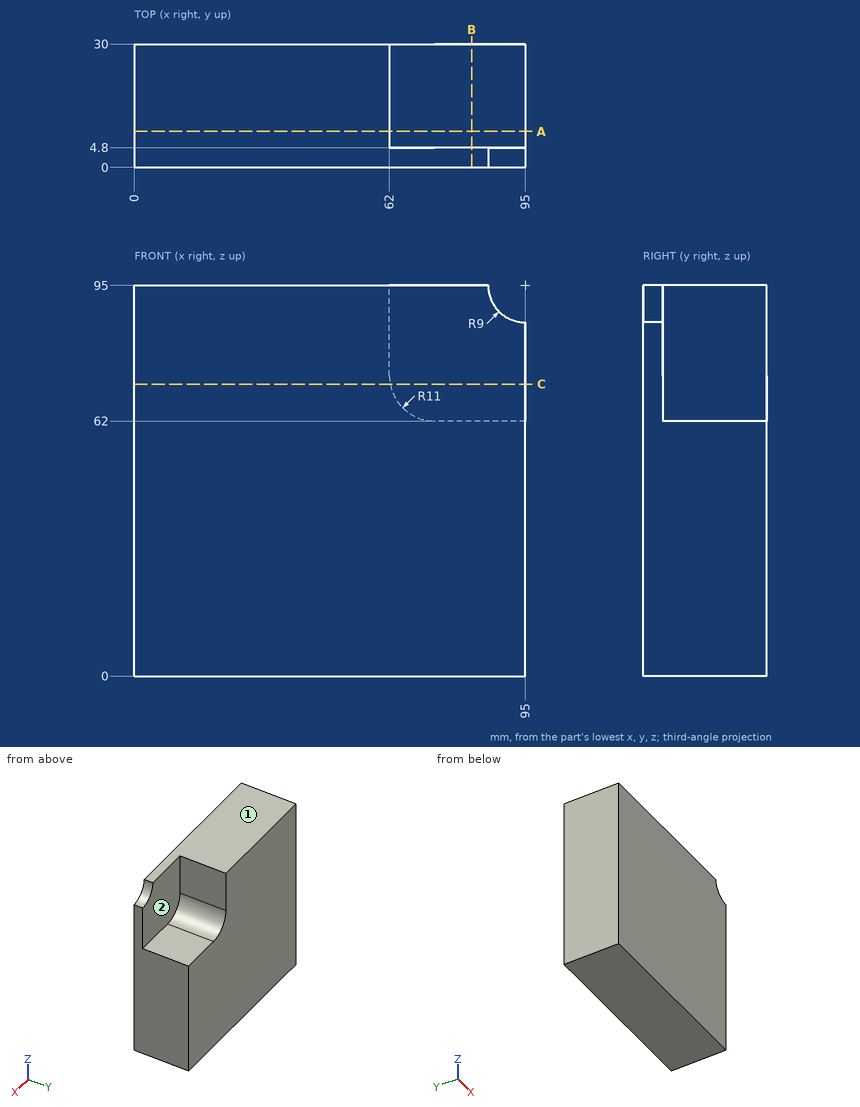
For this review, use the dimensioned drawing (mm, ordinates from the lowest corner) and the shaded views. A direction names the side the tool comes from. Round coordinates to 2 decimals unless told otherwise and drop trailing zeros. Write each loop counter-clockwise with the first axis right and the second up, starting at its lowest first coordinate (ties: lowest second). Pieces come first, ordered by that corner, then holes. Notation, with made-up numbers: M 46,30.25 L 66,30.25 A11 ccw 66,35.25 Z; hole C 1.25,78 d9. An arc over 180 degrees is marked long. Use CSV: the item, a comma, the result in double quotes. Start each with the question number.
(1) We need section B-B, the plane x = 82. State the section outline as (y, z) points.
(2) Tool access review of the marked faces 1 and 2: name each direction out of +Z, -Z, +X, -X, +Y, -Y from which nothing blocks a thin tool from reaching the whole face with its end or side.
(3) For line 1 along X through (y, z) = (22.5, 78.5); line 2 along Z through (x, y) = (66.5, 20), list the stretches that pass through material, from the lowest coordinate up.
(4) Clearance check with flat-ended pins moving along their axes: P1, Ø12, axis at x = 31.5, y = 15, coming from the -Z side; P2, Ø17.5, axis at x = 81.5, y = 17.5, coming from the +Z side; P3, Ø6.5, axis at y = 17, z = 78.5, coming from the +X side. State where each tip first meets the part, or that it passes through.
(5) We need section A-A, the plane y = 8.75. State the section outline as (x, z) points, then the cut area to 3 significant figures.
(6) We need section C-C, the plane z = 71. State the section outline as (x, y) points, then the cut area to 3 significant figures.
Findings:
1,outline,"M 0,0 L 30,0 L 30,62 L 4.8,62 L 4.8,95 L 0,95 Z"
2,face 1,"+Z, +X, -X, +Y, -Y"
2,face 2,"+Z, +X, +Y"
3,line 1,"0 to 62"
3,line 2,"0 to 64.13"
4,P1,"z = 0"
4,P2,"z = 62"
4,P3,"x = 62"
5,outline,"M 0,0 L 95,0 L 95,62 L 73,62 A11 cw 62,73 L 62,95 L 0,95 Z"
5,area,"7,960 mm^2"
6,outline,"M 0,0 L 95,0 L 95,4.8 L 62.18,4.8 L 62.18,30 L 0,30 Z"
6,area,"2,020 mm^2"
